Could you check a few things on this model? Use its own coordinates, in mm. Give positions to 0.01 mm unless a question says otherwise; leave off trailing zeros. Write each loop counter-clockwise with the first axis right and the second up, starting at its lowest first coordinate (ties: lowest second). Pieces come first, ordered by that corner, then holes. Notation, with made-up numbers: (-16.5, -28) - (24.5, -28) arc R23 cw to (24.5, -11) - close; hole circle Ø7 at (51.25, -9.75). An arc over 180 degrees is marked (long way). Use one line per item in the form item = value.
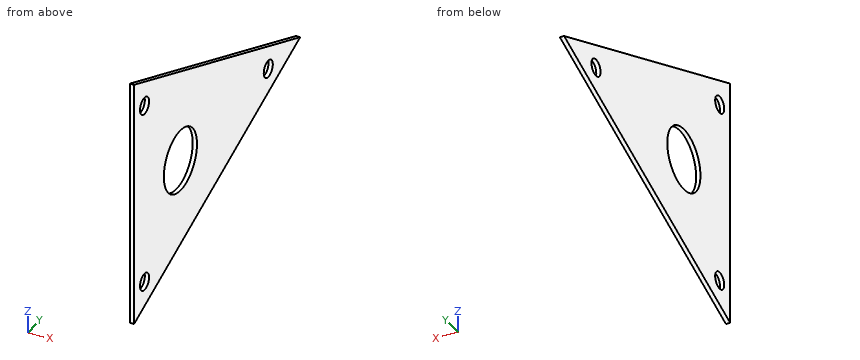
Autodesk Inventor part; units mm, degrees
ref_plane "YZ Plane" through (0, 0, 0) normal (1, 0, 0) x (0, 1, 0)
ref_plane "XZ Plane" through (0, 0, 0) normal (0, 1, 0) x (-1, 0, 0)
ref_plane "XY Plane" through (0, 0, 0) normal (0, 0, 1) x (1, 0, 0)
sketch "Esboço1" plane through (0, 0, 0) normal (1, 0, 0) x (0, 1, 0)
  line L0 (0, 0) -> (0, 43) construction
  line L1 (0, 0) -> (0, -43) construction
  line L2 (0, 0) -> (-40, 0) construction
  line L3 (-40, -43) -> (-40, 44.381)
  line L4 (-40, 0) -> (66, 0) construction
  line L5 (-40, -43) -> (70.202, 1.7046)
  line L6 (70.202, 1.7046) -> (-40, 44.381)
  circle A0 centre (-9.265, 0) radius 11
  line L7 (-326.6157, 155.3746) -> (103.2483, -11.0928)
  dimension "d1" = 43
  dimension "d2" = 43
  dimension "d3" = 40
  dimension "d4" = 106
  dimension "d5" = 22
extrude "Extrusão1" add sketch "Esboço1" along normal blind 1.5
sketch "Esboço2" plane through (0, 0, 0) normal (-1, 0, 0) x (0, 0, 1)
  circle A0 centre (1.7046, 49.0262) radius 3
  circle A1 centre (-31.3462, -33.0501) radius 3
  circle A2 centre (32.9237, -33.0501) radius 3
  point P0 (0, 0)
extrude "Extrusão2" cut sketch "Esboço2" against normal blind 2
sketch "Esboço3" plane through (1.5, 0, 0) normal (1, 0, 0) x (0, 0, -1)
  circle A0 centre (0, -9.265) radius 11
ref_plane "Work Plane1" through (0, 70.202, 1.7046) normal (0, -0.008, 1) x (1, 0, 0)
properties part number "fixação KS traseiro"
1. Imagine slicing it at C-C, the plane z = 0. List the corners of the cut face in (x, y) for me (3 decimals), and give its area (3 significant figures).
Response values:
outline = (0, -40) - (1.5, -40) - (1.5, -20.265) - (0, -20.265) - close; (0, 1.735) - (1.5, 1.735) - (1.5, 46.558) - (0, 46.558) - close; (0, 51.495) - (1.5, 51.495) - (1.5, 66) - (0, 66) - close
area = 119 mm²
2. For pin 1 (3.5 mm diameter, centred on y = 49.03, z = 1.7, fed in from +X), with a flat end and sliding along its axis, tell me the tip position at first contact or that it passes through.
Response values:
pin_1 = through
3. Imagine slicing it at D-D, the plane x = 0.35. List the corners of the cut face in (y, z) for me (3 decimals).
Response values:
outline = (-40, -43) - (70.202, 1.705) - (-40, 44.381) - close; hole circle Ø6 at (-33.05, -31.346); hole circle Ø6 at (-33.05, 32.924); hole circle Ø22 at (-9.265, 0); hole circle Ø6 at (49.026, 1.705)
4. Imagine slicing it at A-A, the plane y = -7.5. List the corners of the cut face in (x, z) for me.
Response values:
outline = (0, -29.82) - (1.5, -29.82) - (1.5, -10.86) - (0, -10.86) - close; (0, 10.86) - (1.5, 10.86) - (1.5, 31.8) - (0, 31.8) - close
5. If I drill on line 1 (Z direction, x = 1, y = -12); line 2 (Y direction, x = 0.1, z = -5.5); line 3 (Y direction, x = 0.45, z = -31), over which ranges is the centre line in solid material (lowest first)? Write a range as from..to.
Response values:
line_1 = -31.64..-10.65, 10.65..33.54
line_2 = -40..-18.79, 0.26..52.44
line_3 = -40..-36.03, -30.07..-10.42
6. Imagine slicing it at B-B, the plane z = -9.5. List the corners of the cut face in (x, y) for me, and give its area (3 significant figures).
Response values:
outline = (0, -40) - (1.5, -40) - (1.5, -14.81) - (0, -14.81) - close; (0, -3.72) - (1.5, -3.72) - (1.5, 42.58) - (0, 42.58) - close
area = 107 mm²
